Autodesk Inventor part; units mm, degrees
ref_plane "YZ Plane" through (0, 0, 0) normal (1, 0, 0) x (0, 1, 0)
ref_plane "XZ Plane" through (0, 0, 0) normal (0, 1, 0) x (-1, 0, 0)
ref_plane "XY Plane" through (0, 0, 0) normal (0, 0, 1) x (1, 0, 0)
sketch "Sketch1" plane through (0, 0, 0) normal (0, 0, 1) x (1, 0, 0)
  circle A0 centre (0, 0) radius 2.4 construction
  line L0 (-0.8, 2.2627) -> (-0.8, 0.8)
  line L1 (-0.8, 0.8) -> (-2.2627, 0.8)
  line L2 (-2.2627, -0.8) -> (-0.8, -0.8)
  line L3 (-0.8, -0.8) -> (-0.8, -2.2627)
  line L4 (0.8, -2.2627) -> (0.8, -0.8)
  line L5 (0.8, -0.8) -> (2.2627, -0.8)
  line L6 (2.2627, 0.8) -> (0.8, 0.8)
  line L7 (0.8, 0.8) -> (0.8, 2.2627)
  arc A1 (0.8, 2.2627) -> (-0.8, 2.2627) centre (0, 0) ccw
  arc A2 (-2.2627, 0.8) -> (-2.2627, -0.8) centre (0, 0) ccw
  arc A3 (-0.8, -2.2627) -> (0.8, -2.2627) centre (0, 0) ccw
  arc A4 (2.2627, -0.8) -> (2.2627, 0.8) centre (0, 0) ccw
  dimension "d0" = 4.8
  dimension "d1" = 1.6
extrude "Extrusion1" add sketch "Sketch1" along normal mid plane 24
sketch "Sketch2" plane through (0, 0, -12) normal (0, 0, -1) x (-1, 0, 0)
  line L0 (0.8, 0.8) -> (0.8, 2.2627)
  arc A0 (0.8, 2.2627) -> (-0.8, 2.2627) centre (0, 0) ccw
  line L1 (-0.8, 2.2627) -> (-0.8, 0.8)
  line L2 (-0.8, 0.8) -> (-2.2627, 0.8)
  arc A1 (-2.2627, 0.8) -> (-2.2627, -0.8) centre (0, 0) ccw
  line L3 (-2.2627, -0.8) -> (-0.8, -0.8)
  line L4 (-0.8, -0.8) -> (-0.8, -2.2627)
  arc A2 (-0.8, -2.2627) -> (0.8, -2.2627) centre (0, 0) ccw
  line L5 (0.8, -2.2627) -> (0.8, -0.8)
  line L6 (0.8, -0.8) -> (2.2627, -0.8)
  arc A3 (2.2627, -0.8) -> (2.2627, 0.8) centre (0, 0) ccw
  line L7 (2.2627, 0.8) -> (0.8, 0.8)
  circle A4 centre (0, 0) radius 3.2
  dimension "d7" = 6.4
extrude "Extrusion2" add sketch "Sketch2" against normal blind 0.8
fillet "Fillet1" radius 0.4 4 edges at (0, 2.4, 12) (-2.4, 0, 12) (0, -2.4, 12) (2.4, 0, 12)
fillet "Fillet1" radius 0.1 2 edges at (3.2, 0, -11.2) (3.2, 0, -12)
equation "\"d0\" = kd"
equation "\"d1\" = axlet"
equation "\"d2\" = 3 * lu"
equation "\"d7\" = tsd"
equation "\"d8\" = tsl"
equation "\"d4\" = tf"
equation "\"d10\" = lf"
properties part number "24316-ReddishBrown" material "ABS Plastic"
CAD build for the part. Positions are in the model's coordinates, mm. A direction names the side the tool comes from. Coordinates: 2 decimals unless noted, no trailing zeros. Write each loop counter-clockwise with the first axis right and the second up, starting at its lowest first coordinate (ties: lowest second). Pieces come first, ordered by that corner, then holes. Notation, with made-up numbers: M 41,63 L 98,63 A18 ccw 98,69 Z; hole C 84,41 d2. An arc over 180 degrees is marked long. Return JSON: item names as keys, results as strings.
Item 1: Slice it at C-C, the plane z = -5.75. Write the cut outline in (x, y), and give its area (3 significant figures).
Findings below:
{"outline": "M -2.26,-0.8 L -0.8,-0.8 L -0.8,-2.26 A2.4 ccw 0.8,-2.26 L 0.8,-0.8 L 2.26,-0.8 A2.4 ccw 2.26,0.8 L 0.8,0.8 L 0.8,2.26 A2.4 ccw -0.8,2.26 L -0.8,0.8 L -2.26,0.8 A2.4 ccw Z", "area": "12.5 mm2"}
Item 2: Slice it at A-A, the plane x = 0. Write the cut outline in (y, z).
Findings below:
{"outline": "M -3.2,-11.9 A0.1 ccw -3.1,-12 L 3.1,-12 A0.1 ccw 3.2,-11.9 L 3.2,-11.3 A0.1 ccw 3.1,-11.2 L 2.4,-11.2 L 2.4,11.6 A0.4 ccw 2,12 L -2,12 A0.4 ccw -2.4,11.6 L -2.4,-11.2 L -3.1,-11.2 A0.1 ccw -3.2,-11.3 Z"}
Item 3: Which spindle directions (+Z, -Z, +X, -X, +Y, -Y) get a long thin tool onto all of the face, cutting with end or side? Do faces 1 (the cylindrical face through (-2.4, 0, 0)), 2 (the cylindrical face through (2.4, 0, 0)), 3 (the flat face through (-0.8, -2, 0)), 4 (the cylindrical face through (0, 2.4, 0)), 5 (the cylindrical face through (0, -2.4, 0)). Say none if no direction does.
Findings below:
{"face 1": "+Z, -X", "face 2": "+Z, +X", "face 3": "+Z, -X, -Y", "face 4": "+Z, +Y", "face 5": "+Z, -Y"}
Item 4: Probe line 1 (X direction, y = 1.25, z = 2.5); line 2 (Z direction, x = 2, y = 1.25). List the from-to ranges inside material, lowest first. Write a range as from..to.
Findings below:
{"line 1": "x = -0.8..0.8", "line 2": "z = -12..-11.2"}
Item 5: Drop flat-ended pins along their axis: pin 1 Ø0.7 at (x, z) = (-1.5, -2) entering from -Y; pin 2 Ø1.6 at (y, z) = (-2, 2.5) entering from -X; pin 3 Ø3 at (x, z) = (0, -5.5) entering from -Y. Give the stop position or say it passes through.
Findings below:
{"pin 1": "stops at y = -0.8", "pin 2": "stops at x = -0.8", "pin 3": "stops at y = -2.4"}
